```python
from build123d import *

# Parameters (mm, degrees)
F0_R          = 36.5
F1_DEPTH      = 16
F5_DEPTH      = 6.3
F5_DEPTH_BACK = 2
F6_COUNT      = 8


with BuildPart() as f1:
    # F0 (on Top) → F1 (new body)
    with BuildSketch(Plane.XY):
        Circle(F0_R)
        with BuildLine():
            ThreePointArc((-3.872983, 1), (0, 4), (3.872983, 1))
            Line((3.872983, 1), (5, 1))
            Line((5, 1), (5, -1))
            Line((5, -1), (3.872983, -1))
            ThreePointArc((3.872983, -1), (0, -4), (-3.872983, -1))
            Line((-3.872983, -1), (-5, -1))
            Line((-5, -1), (-5, 1))
            Line((-5, 1), (-3.872983, 1))
        make_face(mode=Mode.SUBTRACT)
    extrude(amount=F1_DEPTH)


with BuildPart() as f5:
    # F3 (on offset) → F5 (new body, two sides)
    with BuildSketch(Plane.XZ.offset(37)) as f5_sk:
        with BuildLine():
            ThreePointArc((0, 0.375), (5.391689, 2.608311), (7.625, 8))
            ThreePointArc((7.625, 8), (-5.391689, 13.391689), (0, 0.375))
        make_face()
    extrude(amount=-F5_DEPTH)
    extrude(f5_sk.sketch, amount=-F5_DEPTH_BACK)


with BuildPart() as f6_1:
    # F6: instance of F5
    add(f5.part.rotate(Axis((0, 0, 8), (0, 0, 1)), 1 * 360 / F6_COUNT))


with BuildPart() as f6_2:
    # F6: instance of F5
    add(f5.part.rotate(Axis((0, 0, 8), (0, 0, 1)), 2 * 360 / F6_COUNT))


with BuildPart() as f6_3:
    # F6: instance of F5
    add(f5.part.rotate(Axis((0, 0, 8), (0, 0, 1)), 3 * 360 / F6_COUNT))


with BuildPart() as f6_4:
    # F6: instance of F5
    add(f5.part.rotate(Axis((0, 0, 8), (0, 0, 1)), 4 * 360 / F6_COUNT))


with BuildPart() as f6_5:
    # F6: instance of F5
    add(f5.part.rotate(Axis((0, 0, 8), (0, 0, 1)), 5 * 360 / F6_COUNT))


with BuildPart() as f6_6:
    # F6: instance of F5
    add(f5.part.rotate(Axis((0, 0, 8), (0, 0, 1)), 6 * 360 / F6_COUNT))


with BuildPart() as f6_7:
    # F6: instance of F5
    add(f5.part.rotate(Axis((0, 0, 8), (0, 0, 1)), 7 * 360 / F6_COUNT))


with BuildPart() as f1_1:
    add(f1.part)

    # F7: cut F5, F6_1, F6_2, F6_3, F6_4, F6_5, F6_6, F6_7
    add(f5.part, mode=Mode.SUBTRACT)
    add(f6_1.part, mode=Mode.SUBTRACT)
    add(f6_2.part, mode=Mode.SUBTRACT)
    add(f6_3.part, mode=Mode.SUBTRACT)
    add(f6_4.part, mode=Mode.SUBTRACT)
    add(f6_5.part, mode=Mode.SUBTRACT)
    add(f6_6.part, mode=Mode.SUBTRACT)
    add(f6_7.part, mode=Mode.SUBTRACT)


solid = f1_1.part
```
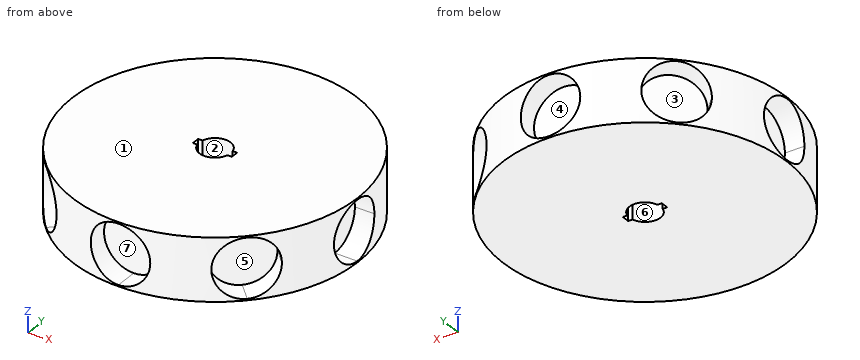
CAD build for the part. Positions are in the model's coordinates, mm. Face numbers are marked on the shaded views. A direction names the side the tool comes from. Round coordinates to 2 decimals unless told otherwise and drop trailing zeros. Loops run counter-clockwise (first coordinate to the right, second up) from the corner with the lowest first, then second, coordinate; pieces in that order, holes last. Notation, with made-up numbers: (11, 88) - (47, 88) arc R23 ccw to (47, 99) - close; hole circle Ø8 at (36, 9.25). An arc over 180 degrees is marked (long way). Return JSON: item names as keys, results as strings. Group by question number.
Q1. Flat gauge pins, fed straight in: pin 1 Ø1.5 at (y, z) = (5.5, 5.5) entering from +X; pin 2 Ø7.5 at (x, z) = (-0.5, 9) entering from +Y; pin 3 Ø2 at (x, z) = (7, 11) entering from +Y. Where does each tip first touch, or does it go through?
Q2. Band-saw the part on C-C on x = 17.5. Give the number of separate pieces and of enclosed holes in the cut face, plus the area to 3 significant figures.
Q3. Two-plate mould, pull along Z, no slides. Class the marked faces 1, 2 and 3: +Z half, -Z half, draft (parallel to the pull), parting line (faces both ways), or undercut.
Q4. Band-saw the part on D-D on y = 14. Give the cut face in (x, z).
Q5. Band-saw the part on A-A on y = -2. Give the cut face in (x, z).
Q6. Tool access for the marked faces 4, 5, 6 and 7: list every direction of +Z, -Z, +X, -X, +Y, -Y with a clear straight run to the whole face (end or side of a thin tool).
Q7. Drill centre lines: line 1 along X through (y, z) = (-18.5, 7.5); line 2 along Z through (x, y) = (34.05, 0) (3 decimals); line 3 along X through (y, z) = (0, 11.5). Where is each one in solid material? Low to high. Write a range as [from, to].
Q8. Band-saw the part on B-B on y = 6. Give the cut face in (x, z), plus the area to 3 significant figures.
Solutions:
{
 "1": {"pin 1": "stops at x = 30.7", "pin 2": "stops at y = 30.7", "pin 3": "stops at y = 35.91"},
 "2": {"separate pieces": "1", "enclosed holes": "2", "area": "994 mm^2"},
 "3": {"face 1": "+Z half", "face 2": "draft", "face 3": "undercut"},
 "4": {"outline": "(-33.71, 0) - (33.71, 0) - (33.71, 16) - (-33.71, 16) - close"},
 "5": {"outline": "(-36.45, 0) - (-3.46, 0) - (-3.46, 16) - (-36.45, 16) - (-36.45, 15.36) - (-30.7, 15.36) - (-30.7, 0.64) - (-36.45, 0.64) - close; (3.46, 0) - (36.45, 0) - (36.45, 0.64) - (30.7, 0.64) - (30.7, 15.36) - (36.45, 15.36) - (36.45, 16) - (3.46, 16) - close"},
 "6": {"face 4": "+Y", "face 5": "none", "face 6": "+Z, -Z", "face 7": "-Y"},
 "7": {"line 1": "x = [-31.46, -29.26], [-24.92, 24.92], [29.26, 31.46]", "line 2": "z = [0, 0.375], [15.625, 16]", "line 3": "x = [-30.7, -5], [5, 30.7]"},
 "8": {"outline": "(-36, 0) - (36, 0) - (36, 3.29) - (30.7, 3.29) - (30.7, 12.71) - (36, 12.71) - (36, 16) - (-36, 16) - (-36, 12.71) - (-30.7, 12.71) - (-30.7, 3.29) - (-36, 3.29) - close", "area": "1,050 mm^2"}
}
